Autodesk Inventor part; units mm, degrees
ref_plane "YZ Plane" through (0, 0, 0) normal (1, 0, 0) x (0, 1, 0)
ref_plane "XZ Plane" through (0, 0, 0) normal (0, 1, 0) x (-1, 0, 0)
ref_plane "XY Plane" through (0, 0, 0) normal (0, 0, 1) x (1, 0, 0)
sketch "Skizze3" plane through (0, 0, 0) normal (0, 0, 1) x (1, 0, 0)
  line L0 (0, 0) -> (0, 8)
  line L1 (0, 8) -> (20, 8)
  line L2 (20, 0) -> (0, 0)
  arc A0 (2.5, 22.25) -> (2.5, 17.25) centre (2.5, 19.75) ccw construction
  arc A1 (17.5, 12.25) -> (17.5, 17.25) centre (17.5, 14.75) ccw construction
  line L3 (17.5, 17.25) -> (2.5, 17.25) construction
  line L4 (2.5, 22.25) -> (17.5, 22.25) construction
  arc A2 (17.5, 22.25) -> (17.5, 27.25) centre (17.5, 24.75) ccw construction
  arc A3 (4.4592, 31.3029) -> (2.5, 27.25) centre (2.5, 29.75) ccw construction
  line L5 (17.5, 27.25) -> (2.5, 27.25) construction
  line L6 (2.5, 12.25) -> (17.5, 12.25) construction
  arc A4 (2.5, 12.25) -> (0.7146, 8) centre (2.5, 9.75) ccw construction
  line L7 (0, 31.5) -> (0, 51.5)
  line L8 (0, 51.5) -> (20, 51.5)
  arc A5 (0, 31.8267) -> (2.5, 26.5) centre (2.5, 29.75) ccw
  line L9 (2.5, 26.5) -> (17.5, 26.5)
  arc A6 (17.5, 23) -> (17.5, 26.5) centre (17.5, 24.75) ccw
  line L10 (17.5, 23) -> (2.5, 23)
  arc A7 (2.5, 23) -> (2.5, 16.5) centre (2.5, 19.75) ccw
  line L11 (2.5, 16.5) -> (17.5, 16.5)
  arc A8 (17.5, 13) -> (17.5, 16.5) centre (17.5, 14.75) ccw
  line L12 (17.5, 13) -> (2.5, 13)
  arc A9 (2.5, 13) -> (0, 7.6733) centre (2.5, 9.75) ccw
  arc A10 (2.5, 31.5) -> (2.5, 28) centre (2.5, 29.75) ccw
  line L13 (2.5, 28) -> (17.5, 28)
  arc A11 (17.5, 21.5) -> (17.5, 28) centre (17.5, 24.75) ccw
  line L14 (17.5, 21.5) -> (2.5, 21.5)
  arc A12 (2.5, 21.5) -> (2.5, 18) centre (2.5, 19.75) ccw
  line L15 (2.5, 18) -> (17.5, 18)
  arc A13 (17.5, 11.5) -> (17.5, 18) centre (17.5, 14.75) ccw
  line L16 (17.5, 11.5) -> (2.5, 11.5)
  arc A14 (2.5, 11.5) -> (2.5, 8) centre (2.5, 9.75) ccw
  line L17 (0, 31.5) -> (20, 31.5)
  line L18 (20, 31.5) -> (20, 31.5)
  line L19 (20, 31.5) -> (20, 41.5)
  line L20 (20, 51.5) -> (20, 41.5)
  line L21 (20, 31.5) -> (45, 31.5)
  line L22 (45, 31.5) -> (45, 41.5)
  line L23 (45, 41.5) -> (20, 41.5)
  line L24 (20, 0) -> (20, 8)
  point P0 (10, 4)
  point P1 (0, 4)
  point P2 (10, 0)
  dimension "d4" = 8
  dimension "d11" = 5
  dimension "d12" = 5
  dimension "d13" = 5
  dimension "d14" = 5
  dimension "d17" = 5
  dimension "d19" = 0.75
  dimension "d20" = 0.75
  dimension "d22" = 20
  dimension "d23" = 20
  dimension "d24" = 10
  dimension "d29" = 25
  dimension "d54" = 20
extrude "Extrusion3" add sketch "Skizze3" along normal blind 18
sketch "Skizze4" plane through (20, 31.5, 0) normal (0, 1, 0) x (1, 0, 0)
  circle A0 centre (16, -9) radius 2
  line L0 (25, 0) -> (25, -18)
  line L1 (25, -18) -> (0, -18)
  line L2 (25, 0) -> (0, 0)
  circle A1 centre (6, -9) radius 2.5
  line L3 (0, 0) -> (0, -18)
  arc A2 (16, -18) -> (16, 0) centre (16, -9) ccw
  line L4 (0, -18) -> (25, -18)
  arc A3 (16, 0) -> (16, -18) centre (16, -9) ccw construction
  circle A4 centre (6, -9) radius 5.25
  point P0 (25, -9)
  point P1 (25, -9)
  point P2 (21, -1.5167)
  dimension "d31" = 4
  dimension "d36" = 5
  dimension "d37" = 6
  dimension "d38" = 10
  dimension "d57" = 10.5
sketch "Skizze6" plane through (0, 51.5, 0) normal (0, 1, 0) x (1, 0, 0)
  circle A0 centre (10, -9) radius 5
  line L0 (20, -18) -> (0, -18)
  line L1 (0, 0) -> (0, -18)
  point P0 (10, -18)
  point P1 (0, -9)
  dimension "d51" = 10
extrude "Extrusion9" cut sketch "Skizze6" against normal through all
extrude "Extrusion6" cut sketch "Skizze4" along normal blind 18 contours L0 A2 L2 | L0 L1 A2 | A1
extrude "Extrusion7" add sketch "Skizze4" against normal blind 10 contours A0
hole "Bohrung1" at (10, 4, 0) direction (0, 0, 1) diameter 2.459 end up to surface
fillet "Rundung3" radius 2 8 edges at (0, 51.5, 9) (20, 51.5, 9) (20, 41.5, 9) (20, 0, 9) (20, 8, 9) (0, 0, 9) (0, 7.6733, 9) (0, 31.8267, 9)
sketch "Skizze7" plane through (0, 0, 18) normal (0, 0, 1) x (1, 0, 0)
  line L0 (20, 43.5) -> (20, 49.5)
  line L1 (20, 43.5) -> (50, 43.5)
  line L2 (50, 43.5) -> (50, 0)
  line L3 (50, 0) -> (20, 0)
  line L4 (20, 0) -> (20, 43.5)
  line L5 (2, 0) -> (18, 0)
  point P0 (0, 0)
  point P1 (35, 0)
  dimension "d68" = 30
extrude "Extrusion11" cut sketch "Skizze7" against normal through all
fillet "Rundung4" radius 2 1 edges at (20, 31.5, 9)
equation "\"d12\" = d11"
properties part number "BT505_trajan20_22"
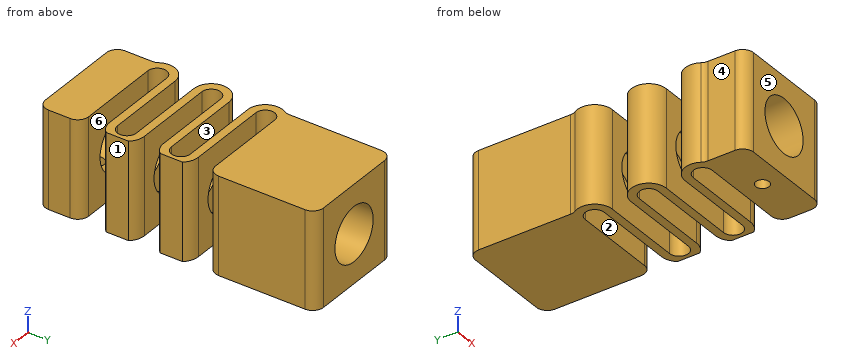
Could you check a few things on this model? Use its own coordinates, in mm. Face numbers are marked on the shaded views. A direction names the side the tool comes from. Round coordinates to 2 decimals unless told otherwise and drop trailing zeros. Write each loop counter-clockwise with the first axis right and the second up, starting at its lowest first coordinate (ties: lowest second). Pieces come first, ordered by that corner, then holes. Notation, with made-up numbers: M -8.5,-30.75 L 43.5,-30.75 A12 cw 43.5,-24.75 Z; hole C 12.25,22 d10. An arc over 180 degrees is marked long. Write each question's results on one line, items separated by ' | '. Start each with the question number.
1. Thinking about a two-plate mould opening in Y: for the marked faces 4, 5 and 6, which applies, +Y half, -Y half, draft (parallel to the pull), parting line (faces both ways), or undercut?
2. Imagine slicing it at C-C on y = 9.75. List the corners of the cut face in (x, z) for me, and give its area (3 significant figures).
3. Imagine slicing it at B-B on x = 7. Count the separate pieces of the cut face and the enclosed holes in it, and give its area (3 significant figures).
4. I'm going to push flat-ended pins straight in: pin 1 Ø7.5 at (x, z) = (10.5, 7.5) entering from -Y; pin 2 Ø8.5 at (y, z) = (37, 11.5) entering from -X; pin 3 Ø2 at (y, z) = (8.5, 12.5) entering from +X. Where does each tip first touch, or does it pass through?
5. On a 3-axis mill with a long thin cutter (end or side, diameter ignored), from which of +Z, -Z, +X, -X, +Y, -Y can I reach the whole of each face in a straight line? I mean the marked faces 1, 2 and 3. Say none if no direction works.
6. I need wall thicknesses on L1, parallel to Y at x = 3.75, z = 13; L2, parallel to Z at x = 10, y = 12.55; L3, parallel to X at y = 4.25, z = 9. Which ranges of each line are inside material? Lowest first, please. Write a range as from..to.
7. Imagine slicing it at A-A on y = 38. List the corners of the cut face in (x, z) for me.
Result sheet:
1) face 4: draft | face 5: -Y half | face 6: undercut
2) outline: M -0.75,0 L 0.75,0 L 0.75,18 L -0.75,18 Z | area: 27.0 mm^2
3) separate pieces: 12 | enclosed holes: 0 | area: 340 mm^2
4) pin 1: stops at y = 0 | pin 2: stops at x = 0 | pin 3: stops at x = 19.32
5) face 1: +Z, -Z, +X, +Y, -Y | face 2: +Z, -Z, +X | face 3: +Z, -Z, -X
6) L1: y = 0..8, 11.5..13, 16.5..18, 21.5..23, 26.5..28, 31.5..51.5 | L2: z = 0..4, 14..18 | L3: x = 0..5, 15..20
7) outline: M 0,0 L 20,0 L 20,18 L 0,18 Z; hole C 10,9 d10
